The listing builds one solid part. Answer for the finished solid, in the listing's coordinates (mm). Face numbers are marked on the shaded views. Give positions to 0.01 mm unless a question says otherwise; leave off trailing zeros. Write each loop counter-clockwise with the first axis right and the second up, starting at its lowest first coordinate (ties: lowest second). Pieces come first, ordered by that corner, then holes.
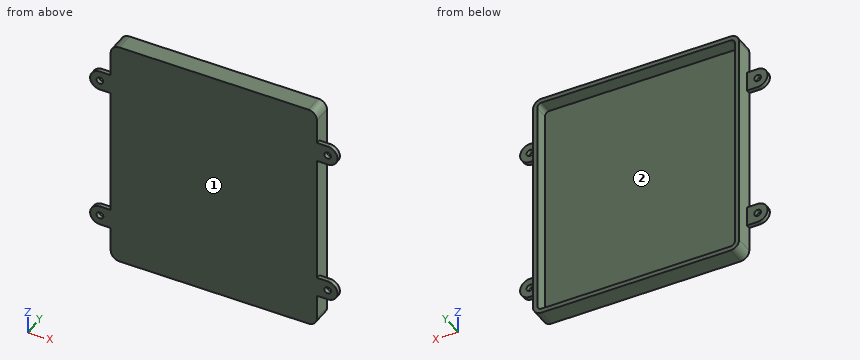
```python
from build123d import *

# Parameters (mm, degrees)
SALIENTE_EXTRUIR1_DEPTH = 8.5
SALIENTE_EXTRUIR2_DEPTH = 2
CROQUIS3_R              = 1.55
SALIENTE_EXTRUIR3_DEPTH = 2


with BuildPart() as part:
    # Croquis1 → Saliente-Extruir1 (new body)
    with BuildSketch(Plane(origin=(0, 0, 0), x_dir=(1, 0, 0), z_dir=(0, 1, 0))):
        with BuildLine():
            Line((-47.75, 50.1), (-47.75, -50.1))
            ThreePointArc((-47.75, -50.1), (-46.578427125, -52.928427125), (-43.75, -54.1))
            Line((-43.75, -54.1), (43.75, -54.1))
            ThreePointArc((43.75, -54.1), (46.578427125, -52.928427125), (47.75, -50.1))
            Line((47.75, -50.1), (47.75, 50.1))
            ThreePointArc((47.75, 50.1), (46.578427125, 52.928427125), (43.75, 54.1))
            Line((43.75, 54.1), (-43.75, 54.1))
            ThreePointArc((-43.75, 54.1), (-46.578427125, 52.928427125), (-47.75, 50.1))
        make_face()
        with BuildLine():
            Line((-43.75, 52.1), (43.75, 52.1))
            ThreePointArc((43.75, 52.1), (45.164213562, 51.514213562), (45.75, 50.1))
            Line((45.75, 50.1), (45.75, -50.1))
            ThreePointArc((45.75, -50.1), (45.164213562, -51.514213562), (43.75, -52.1))
            Line((43.75, -52.1), (-43.75, -52.1))
            ThreePointArc((-43.75, -52.1), (-45.164213562, -51.514213562), (-45.75, -50.1))
            Line((-45.75, -50.1), (-45.75, 50.1))
            ThreePointArc((-45.75, 50.1), (-45.164213562, 51.514213562), (-43.75, 52.1))
        make_face(mode=Mode.SUBTRACT)
    extrude(amount=SALIENTE_EXTRUIR1_DEPTH)

    # Croquis2 → Saliente-Extruir2 (add)
    with BuildSketch(Plane(origin=(0, 0, 0), x_dir=(1, 0, 0), z_dir=(0, 1, 0))):
        with BuildLine():
            Line((43.75, 54.1), (-43.75, 54.1))
            ThreePointArc((-43.75, 54.1), (-46.578427125, 52.928427125), (-47.75, 50.1))
            Line((-47.75, 50.1), (-47.75, -50.1))
            ThreePointArc((-47.75, -50.1), (-46.578427125, -52.928427125), (-43.75, -54.1))
            Line((-43.75, -54.1), (43.75, -54.1))
            ThreePointArc((43.75, -54.1), (46.578427125, -52.928427125), (47.75, -50.1))
            Line((47.75, -50.1), (47.75, 50.1))
            ThreePointArc((47.75, 50.1), (46.578427125, 52.928427125), (43.75, 54.1))
        make_face()
    extrude(amount=SALIENTE_EXTRUIR2_DEPTH)

    # Croquis3 → Saliente-Extruir3 (add)
    with BuildSketch(Plane(origin=(0, 0, 0), x_dir=(1, 0, 0), z_dir=(0, 1, 0))):
        with BuildLine():
            Line((-52.75, 38.65), (-47.75, 38.65))
            Line((-47.75, 38.65), (-47.75, 50.1))
            ThreePointArc((-47.75, 50.1), (-46.578427125, 52.928427125), (-43.75, 54.1))
            Line((-43.75, 54.1), (43.75, 54.1))
            ThreePointArc((43.75, 54.1), (46.578427125, 52.928427125), (47.75, 50.1))
            Line((47.75, 50.1), (47.75, 38.65))
            Line((47.75, 38.65), (52.75, 38.65))
            ThreePointArc((52.75, 38.65), (57.3, 34.1), (52.75, 29.55))
            Line((52.75, 29.55), (47.75, 29.55))
            Line((47.75, 29.55), (47.75, -29.55))
            Line((47.75, -29.55), (52.75, -29.55))
            ThreePointArc((52.75, -29.55), (57.3, -34.1), (52.75, -38.65))
            Line((52.75, -38.65), (47.75, -38.65))
            Line((47.75, -38.65), (47.75, -50.1))
            ThreePointArc((47.75, -50.1), (46.578427125, -52.928427125), (43.75, -54.1))
            Line((43.75, -54.1), (-43.75, -54.1))
            ThreePointArc((-43.75, -54.1), (-46.578427125, -52.928427125), (-47.75, -50.1))
            Line((-47.75, -50.1), (-47.75, -38.65))
            Line((-47.75, -38.65), (-52.75, -38.65))
            ThreePointArc((-52.75, -38.65), (-57.3, -34.1), (-52.75, -29.55))
            Line((-52.75, -29.55), (-47.75, -29.55))
            Line((-47.75, -29.55), (-47.75, 29.55))
            Line((-47.75, 29.55), (-52.75, 29.55))
            ThreePointArc((-52.75, 29.55), (-57.3, 34.1), (-52.75, 38.65))
        make_face()
        with Locations((-52.75, 34.1)):
            Circle(CROQUIS3_R, mode=Mode.SUBTRACT)
        with Locations((52.75, 34.1)):
            Circle(CROQUIS3_R, mode=Mode.SUBTRACT)
        with Locations((52.75, -34.1)):
            Circle(CROQUIS3_R, mode=Mode.SUBTRACT)
        with Locations((-52.75, -34.1)):
            Circle(CROQUIS3_R, mode=Mode.SUBTRACT)
    extrude(amount=SALIENTE_EXTRUIR3_DEPTH)


solid = part.part
```
Item 1: A cutting plane is placed at A-A, the plane z = 34.1. Give the vertices of the cut face in (x, y), plus the area to 3 significant figures.
Conclusion:
outline: (-57.3, 0) - (-54.3, 0) - (-54.3, 2) - (-57.3, 2) - close; (-51.2, 0) - (51.2, 0) - (51.2, 2) - (47.75, 2) - (47.75, 8.5) - (45.75, 8.5) - (45.75, 2) - (-45.75, 2) - (-45.75, 8.5) - (-47.75, 8.5) - (-47.75, 2) - (-51.2, 2) - close; (54.3, 0) - (57.3, 0) - (57.3, 2) - (54.3, 2) - close
area: 243 mm2
Item 2: Each of these flat-tipped pins is pushed along its axis until it touches: P1, Ø2, axis at x = 50.5, y = 1.5, coming from the +Z side; P2, Ø8, axis at x = 15.5, z = 36.5, coming from the -Y side; P3, Ø2, axis at x = 50.5, y = 1.5, coming from the -Z side; P4, Ø4.5, axis at x = -53, z = -34, coming from the +Y side. Where does it stop, or does it pass through?
Conclusion:
P1: stops at z = 38.65
P2: stops at y = 0
P3: stops at z = -38.65
P4: stops at y = 2
Item 3: A cutting plane is placed at C-C, the plane x = 17. Give the vertices of the cut face in (y, z).
Conclusion:
outline: (0, -54.1) - (8.5, -54.1) - (8.5, -52.1) - (2, -52.1) - (2, 52.1) - (8.5, 52.1) - (8.5, 54.1) - (0, 54.1) - close
Item 4: Determine the mould class of the marked faces 1 and 2 for opening direction Z: pulls with the +Z half, pulls with the -Z half, needs draft (parallel to the pull), parting line crosses it, or undercut.
Conclusion:
face 1: needs draft
face 2: undercut
Item 5: Consider probe 1 along X at (y, z) = (0.7, -34.1); probe 2 along Z at (x, y) = (-52.75, 1.1); probe 3 along X at (y, z) = (8, 40.5). Determine where each line is inside the solid, lowest interval first.
Conclusion:
probe 1: x = -57.3 to -54.3, -51.2 to 51.2, 54.3 to 57.3
probe 2: z = -38.65 to -35.65, -32.55 to -29.55, 29.55 to 32.55, 35.65 to 38.65
probe 3: x = -47.75 to -45.75, 45.75 to 47.75
Item 6: A cutting plane is placed at B-B, the plane z = 15. Give the vertices of the cut face in (x, y), plus the area to 3 significant figures.
Conclusion:
outline: (-47.75, 0) - (47.75, 0) - (47.75, 8.5) - (45.75, 8.5) - (45.75, 2) - (-45.75, 2) - (-45.75, 8.5) - (-47.75, 8.5) - close
area: 217 mm2
